Verification items for the finished model (mm, model axes). Face numbers are marked on the shaded views. A direction names the side the tool comes from. Round coordinates to 2 decimals unless told otherwise and drop trailing zeros. Write each loop counter-clockwise with the first axis right and the second up, starting at its lowest first coordinate (ties: lowest second). Pieces come first, ordered by that corner, then holes. Notation, with made-up numbers: (14.25, 50.25) -> (36.25, 50.25) arc R23 ccw to (36.25, 80.25) -> close; hole circle Ø1 at (-10.75, 83.5). An arc over 180 degrees is marked (long way). Answer as a JSON object with one key per item and string values. Group by question number.
(1) Sectioned sample at A-A on x = 0. Record the cut outline in (y, z), and give its area (3 significant figures).
(2) Draft check along X on the marked faces 1, 2 and 3. Enter one of: released by +X, released by -X, zero draft, split by the parting line, or undercut.
(3) Set-up check for the marked faces 4 and 5: record each of +Z, -Z, +X, -X, +Y, -Y from which the full face is reachable in a straight line by a thin tool's end or side.
(4) Scan lines: L1, parallel to X at y = 3.25, z = 0.2; L2, parallel to Y at x = 0, z = 0.45; L3, parallel to Y at x = 3, z = 0.65. Record each from-to range of solid material in increasing order. Write a range as from..to.
(5) Gauge pin test, flat ends, axial feed: pin 1 Ø8 at (x, y) = (9, 1.5) entering from -Z; pin 2 Ø5 at (x, y) = (2, -3.5) entering from -Z; pin 3 Ø3.5 at (x, y) = (0, 0) entering from +Z; pin 4 Ø0.6 at (x, z) = (7.5, 1.5) entering from +Y. Record the tip position at first contact, or that the pin passes through.
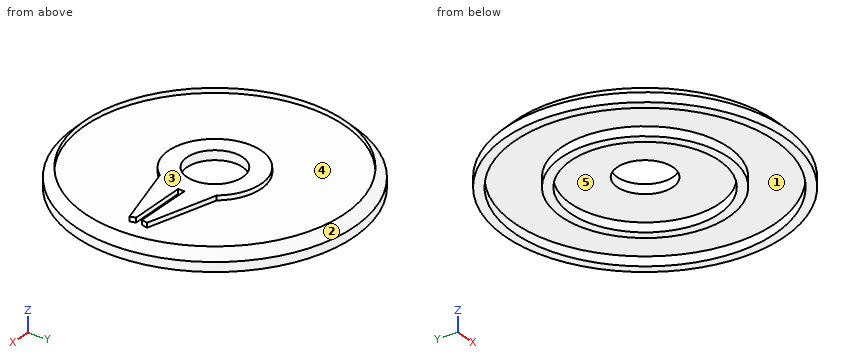
```python
from build123d import *

# Parameters (mm, degrees)
F0_R      = 15
F1_DEPTH  = 2
F2_R      = 14
F3_DEPTH  = 1
F4_SIZE   = 1
F5_R      = 4
F6_DEPTH  = 25
F8_R      = 14
F9_DEPTH  = 0.5
F10_R     = 4
F10_R_2   = 3
F11_DEPTH = 1
F12_R     = 9
F12_R_2   = 8
F13_DEPTH = 1


with BuildPart() as f1:
    # F0 (on Top) → F1 (new body)
    with BuildSketch(Plane.XY):
        Circle(F0_R)
    extrude(amount=F1_DEPTH)

    # F2 (on face) → F3 (cut)
    with BuildSketch(Plane(origin=(0, 0, 0), x_dir=(1, 0, 0), z_dir=(0, 0, -1))):
        Circle(F2_R)
    extrude(amount=-F3_DEPTH, mode=Mode.SUBTRACT)

    # F4
    f4_edges = [f1.edges().sort_by_distance(p)[0] for p in [
        (-15, 0, 2),
    ]]
    chamfer(f4_edges, length=F4_SIZE)

    # F5 (on face) → F6 (cut)
    with BuildSketch(Plane.XY.offset(2)):
        Circle(F5_R)
    extrude(amount=-F6_DEPTH, mode=Mode.SUBTRACT)

    # F8 (on face) → F9 (cut)
    with BuildSketch(Plane.XY.offset(2)):
        Circle(F8_R)
        with BuildLine():
            ThreePointArc((4.9880774736, 0.3450842174), (4.9970184795, 0.1726450576), (5, 0))
            ThreePointArc((5, 0), (4.9970184795, -0.1726450576), (4.9880774736, -0.3450842174))
            Line((4.9880774736, -0.3450842174), (11.2447906452, -0.3450842174))
            Line((11.2447906452, -0.3450842174), (11.4114703611, -0.9285551496))
            Line((11.4114703611, -0.9285551496), (3.955437905, -3.0585145054))
            ThreePointArc((3.955437905, -3.0585145054), (-4.9999982746, 0.00415382), (3.9605142509, 3.0519382151))
            Line((3.9605142509, 3.0519382151), (11.4327203482, 0.956684351))
            Line((11.4327203482, 0.956684351), (11.2488549203, 0.3009736538))
            Line((11.2488549203, 0.3009736538), (4.9880774736, 0.3450842174))
        make_face(mode=Mode.SUBTRACT)
    extrude(amount=-F9_DEPTH, mode=Mode.SUBTRACT)

    # F10 (on face) → F11 (join)
    with BuildSketch(Plane.XY.offset(2)):
        Circle(F10_R)
        Circle(F10_R_2, mode=Mode.SUBTRACT)
    extrude(amount=-F11_DEPTH)

    # F12 (on face) → F13 (join)
    with BuildSketch(Plane(origin=(0, 0, 1), x_dir=(1, 0, 0), z_dir=(0, 0, -1))):
        Circle(F12_R)
        Circle(F12_R_2, mode=Mode.SUBTRACT)
    extrude(amount=F13_DEPTH)


solid = f1.part
```
Computed values:
{
 "1": {"outline": "(-15, 0) -> (-14, 0) -> (-14, 1) -> (-9, 1) -> (-9, 0) -> (-8, 0) -> (-8, 1) -> (-3, 1) -> (-3, 2) -> (-5, 2) -> (-5, 1.5) -> (-14, 1.5) -> (-14, 2) -> (-15, 1) -> close; (3, 1) -> (8, 1) -> (8, 0) -> (9, 0) -> (9, 1) -> (14, 1) -> (14, 0) -> (15, 0) -> (15, 1) -> (14, 2) -> (14, 1.5) -> (5, 1.5) -> (5, 2) -> (3, 2) -> close", "area": "18.0 mm2"},
 "2": {"face 1": "undercut", "face 2": "split by the parting line", "face 3": "zero draft"},
 "3": {"face 4": "+Z", "face 5": "-Z"},
 "4": {"L1": "-14.64..-13.62, -8.39..-7.31, 7.31..8.39, 13.62..14.64", "L2": "-15..-14, -9..-8, 8..9, 14..15", "L3": "-14.7..-13.67, -8.49..-7.42, 7.42..8.49, 13.67..14.7"},
 "5": {"pin 1": "z = 0", "pin 2": "z = 1", "pin 3": "through", "pin 4": "y = 12.8"}
}
